Read the model definition and answer for the solid it produces. Units are mm, in the model's axes. Face numbers are marked on the shaded views. A direction names the side the tool comes from. Give positions to 0.01 mm unless a question says otherwise; leave off trailing zeros. Order: outer loops, then holes, each group sorted by start corner. A loop starts at its lowest first (then second) coordinate and runs counter-clockwise, first axis right, second up. Notation, with made-up numbers: (38.25, 86.5) - (67.25, 86.5) arc R18 ccw to (67.25, 93.5) - close; hole circle Ø4 at (64, -30). An arc over 180 degrees is marked (long way). Return JSON: item names as keys, results as strings.
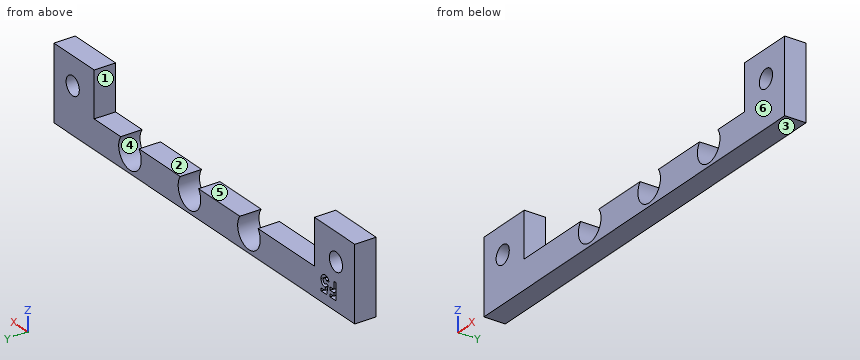
```python
from build123d import *

# Parameters (mm, degrees)
BOSS_EXTRUDE1_OUTLINE_R = 1.75
BOSS_EXTRUDE1_DEPTH     = 4
CUT_EXTRUDE1_DEPTH      = 1


# Read off the part's stored shape, not the designer's step: Boss-Extrude1
with BuildPart() as part:
    # Boss-Extrude1 outline → Boss-Extrude1 (new body)
    with BuildSketch(Plane(origin=(0, 0, 0), x_dir=(1, 0, 0), z_dir=(0, 1, 0))):
        with BuildLine():
            Line((24.976474615, -10.33744254), (35.92307775, -10.33744254))
            ThreePointArc((35.92307775, -10.33744254), (38.359776182, -5.587442326), (40.796474615, -10.33744254))
            Line((40.796474615, -10.33744254), (47.859776182, -10.33744254))
            Line((47.859776182, -10.33744254), (47.859776182, -18.81631662))
            Line((47.859776182, -18.81631662), (58.584776182, -18.81631662))
            Line((58.584776182, -18.81631662), (58.584776182, -4.977921711))
            Line((58.584776182, -4.977921711), (-21.415223818, -4.977921711))
            Line((-21.415223818, -4.977921711), (-21.415223818, -18.81631662))
            Line((-21.415223818, -18.81631662), (-10.690223818, -18.81631662))
            Line((-10.690223818, -18.81631662), (-10.690223818, -10.33744254))
            Line((-10.690223818, -10.33744254), (4.28307775, -10.33744254))
            ThreePointArc((4.28307775, -10.33744254), (6.719776183, -5.587442326), (9.156474615, -10.33744254))
            Line((9.156474615, -10.33744254), (20.10307775, -10.33744254))
            ThreePointArc((20.10307775, -10.33744254), (22.539776182, -5.587442326), (24.976474615, -10.33744254))
        make_face()
        with Locations((-16.415223818, -13.587442433)):
            Circle(BOSS_EXTRUDE1_OUTLINE_R, mode=Mode.SUBTRACT)
        with Locations((53.584776182, -13.587442433)):
            Circle(BOSS_EXTRUDE1_OUTLINE_R, mode=Mode.SUBTRACT)
    extrude(amount=BOSS_EXTRUDE1_DEPTH)

    # Sketch2 → Cut-Extrude1 (cut)
    with BuildSketch(Plane(origin=(0, 4, 0), x_dir=(1, 0, 0), z_dir=(0, 1, 0))):
        Polygon((-16.41198232, -6.812466594), (-14.865187448, -6.812466594), (-14.865187448, -7.382338389), (-15.842110525, -7.382338389), (-15.842110525, -7.992915312), (-14.865187448, -7.992915312), (-14.865187448, -8.562787107), (-15.842110525, -8.562787107), (-15.842110525, -9.987466594), (-16.41198232, -9.987466594), align=None)
        with BuildLine():
            Line((-13.949958082, -6.812466594), (-12.504290013, -6.812466594))
            Line((-12.504290013, -6.812466594), (-12.504290013, -7.341633261))
            Line((-12.504290013, -7.341633261), (-13.498385565, -7.341633261))
            Line((-13.498385565, -7.341633261), (-13.622409003, -7.942033902))
            add(Edge.make_bspline(
                [(-13.622409003, -7.942033902), (-13.605509034, -7.937327047), (-13.572178824, -7.928044162), (-13.52196682, -7.918734604), (-13.473304391, -7.912700444), (-13.441372402, -7.911895568), (-13.425879556, -7.911505055)],
                knots=[0, 0, 0, 0, 1.05461699, 2.079921384, 3.068411212, 4, 4, 4, 4], degree=3))
            add(Edge.make_bspline(
                [(-13.425879556, -7.911505055), (-13.392119021, -7.912278658), (-13.325569569, -7.913803601), (-13.228216166, -7.928280275), (-13.134994532, -7.951080599), (-13.046189934, -7.983598566), (-12.961889124, -8.025921539), (-12.881989912, -8.077120472), (-12.806394235, -8.137285289), (-12.73644499, -8.20645366), (-12.672172703, -8.282402096), (-12.616291615, -8.364548366), (-12.568565678, -8.451721144), (-12.530606118, -8.544462294), (-12.500645197, -8.642189339), (-12.478994766, -8.744964906), (-12.466191785, -8.852910799), (-12.464465382, -8.926554564), (-12.463584884, -8.96411423)],
                knots=[0, 0, 0, 0, 1.01440847, 1.999622559, 2.951875003, 3.895578053, 4.836219714, 5.782137149, 6.743708247, 7.735272588, 8.734977101, 9.730283169, 10.717124674, 11.717316708, 12.737475749, 13.78628267, 14.87096371, 16, 16, 16, 16], degree=3))
            add(Edge.make_bspline(
                [(-12.463584884, -8.96411423), (-12.464660866, -9.002100285), (-12.466784093, -9.077057875), (-12.480636202, -9.187272048), (-12.505085424, -9.292832343), (-12.538668877, -9.394021345), (-12.582912926, -9.490095338), (-12.63612245, -9.582049577), (-12.699197079, -9.669201514), (-12.771517834, -9.750657738), (-12.850139982, -9.82511029), (-12.93385401, -9.890606342), (-13.022071802, -9.94572074), (-13.114795487, -9.990262491), (-13.211493079, -10.025503132), (-13.312193927, -10.051156636), (-13.417387424, -10.065867495), (-13.488800141, -10.067862709), (-13.525098306, -10.06887685)],
                knots=[0, 0, 0, 0, 1.06808661, 2.107647099, 3.116961351, 4.110378221, 5.100014249, 6.085620622, 7.093190682, 8.119403071, 9.144090782, 10.133780668, 11.103064255, 12.062861538, 13.020824475, 13.992378307, 14.979551724, 16, 16, 16, 16], degree=3))
            add(Edge.make_bspline(
                [(-13.525098306, -10.06887685), (-13.557558674, -10.068047219), (-13.621577314, -10.066411014), (-13.715873961, -10.056354031), (-13.806786399, -10.038573192), (-13.893831984, -10.012839713), (-13.97792658, -9.981167676), (-14.058098031, -9.941555807), (-14.134786891, -9.894758372), (-14.207775393, -9.841629423), (-14.275877579, -9.781781722), (-14.338034038, -9.716268103), (-14.394621073, -9.645914331), (-14.444427811, -9.569852456), (-14.487298122, -9.488194854), (-14.525316388, -9.40190388), (-14.556434719, -9.310078379), (-14.572226377, -9.24641984), (-14.580251551, -9.214069158)],
                knots=[0, 0, 0, 0, 1.054957082, 2.080596141, 3.077793124, 4.061112343, 5.027190972, 5.994718051, 6.962465889, 7.943658696, 8.924948258, 9.904494768, 10.875059, 11.855380583, 12.854004648, 13.869083016, 14.917087635, 16, 16, 16, 16], degree=3))
            Line((-14.580251551, -9.214069158), (-13.9289695, -9.214069158))
            add(Edge.make_bspline(
                [(-13.9289695, -9.214069158), (-13.917064048, -9.236486864), (-13.893927162, -9.280053116), (-13.849915688, -9.337893862), (-13.800647638, -9.387217966), (-13.746567435, -9.428507334), (-13.687324675, -9.459440626), (-13.625333386, -9.482899003), (-13.559814799, -9.496454731), (-13.515193749, -9.498149331), (-13.492661407, -9.499005055)],
                knots=[0, 0, 0, 0, 1.104910296, 2.147267069, 3.153527244, 4.136738762, 5.099945312, 6.05603338, 7.018353, 8, 8, 8, 8], degree=3))
            add(Edge.make_bspline(
                [(-13.492661407, -9.499005055), (-13.476956667, -9.49841417), (-13.446057326, -9.497251594), (-13.400532034, -9.491101274), (-13.357076143, -9.479452707), (-13.315366568, -9.463322149), (-13.275291268, -9.443205522), (-13.237424734, -9.417809591), (-13.201108159, -9.388577933), (-13.166894426, -9.355034506), (-13.135906647, -9.317641387), (-13.108733754, -9.277459932), (-13.08443744, -9.235382981), (-13.066440789, -9.189743761), (-13.051703054, -9.141905074), (-13.040849589, -9.09150606), (-13.03436342, -9.038487855), (-13.033762974, -9.002293813), (-13.033456679, -8.983830777)],
                knots=[0, 0, 0, 0, 0.978869489, 1.925942215, 2.855067702, 3.774946051, 4.70828698, 5.642468714, 6.60995405, 7.609372294, 8.622401667, 9.629904756, 10.629323, 11.642352373, 12.678539694, 13.745912462, 14.850161547, 16, 16, 16, 16], degree=3))
            add(Edge.make_bspline(
                [(-13.033456679, -8.983830777), (-13.03381217, -8.965796309), (-13.034504141, -8.930691779), (-13.040228266, -8.879145756), (-13.050468615, -8.830237908), (-13.064421178, -8.783593638), (-13.082282125, -8.739496193), (-13.104109396, -8.697683084), (-13.129996239, -8.65836566), (-13.160081636, -8.622344386), (-13.192164393, -8.589304649), (-13.226631584, -8.560408358), (-13.263172677, -8.536426443), (-13.300652202, -8.515489534), (-13.340566208, -8.500252107), (-13.382017188, -8.489758654), (-13.424961552, -8.48205898), (-13.454252971, -8.481606596), (-13.469128755, -8.48137685)],
                knots=[0, 0, 0, 0, 1.166249705, 2.270133367, 3.348514167, 4.393962215, 5.415026464, 6.420877785, 7.440098956, 8.453121383, 9.451844239, 10.415694839, 11.355045125, 12.27538808, 13.187007209, 14.108269027, 15.039275622, 16, 16, 16, 16], degree=3))
            add(Edge.make_bspline(
                [(-13.469128755, -8.48137685), (-13.485287313, -8.481989978), (-13.51767253, -8.483218817), (-13.565788856, -8.493217552), (-13.613325034, -8.509399257), (-13.660545412, -8.531724482), (-13.706981248, -8.560941158), (-13.753858004, -8.59520897), (-13.799606617, -8.637017798), (-13.828694857, -8.668157109), (-13.843743138, -8.684266474)],
                knots=[0, 0, 0, 0, 0.88288272, 1.769486374, 2.674910571, 3.623812639, 4.617874466, 5.670434592, 6.794841017, 8, 8, 8, 8], degree=3))
            Line((-13.843743138, -8.684266474), (-14.323300429, -8.574235424))
            Line((-14.323300429, -8.574235424), (-13.949958082, -6.812466594))
        make_face()
    extrude(amount=-CUT_EXTRUDE1_DEPTH, mode=Mode.SUBTRACT)


solid = part.part
```
Q1. Given pin 1 (2 mm diameter, centred on x = 16.5, y = 2.5, fed in from +Z); pin 2 (5.5 mm diameter, centred on x = 38.36, z = 8.59, fed in from -Y), each flat-ended and moving along its own axis, determine where each tip first touches the part or whether it passes through.
Values:
{"pin 1": "stops at z = 10.34", "pin 2": "passes through"}
Q2. Determine the mould class of the marked faces 1, 2, 3 and 4 for opening direction Z: released by +Z, released by -Z, zero draft, split by the parting line, or undercut.
Values:
{"face 1": "zero draft", "face 2": "released by +Z", "face 3": "released by -Z", "face 4": "undercut"}
Q3. A cutting plane is placed at A-A (x = 28.5). Write down the section's boundary in (y, z), and give its area (3 significant figures).
Values:
{"outline": "(0, 4.98) - (4, 4.98) - (4, 10.34) - (0, 10.34) - close", "area": "21.4 mm²"}
Q4. For the marked faces 5 and 6, determine the directions among +Z, -Z, +X, -X, +Y, -Y from which every point of the face is accessible in a straight line to the end or side of a thin tool.
Values:
{"face 5": "+Z, +Y, -Y", "face 6": "+Z, -Z, +X, -X, -Y"}
Q5. A cutting plane is placed at B-B (y = 1.85). Write down the section's boundary in (x, z).
Values:
{"outline": "(-21.42, 4.98) - (58.58, 4.98) - (58.58, 18.82) - (47.86, 18.82) - (47.86, 10.34) - (40.8, 10.34) arc R3 cw (long way) to (35.92, 10.34) - (24.98, 10.34) arc R3 cw (long way) to (20.1, 10.34) - (9.16, 10.34) arc R3 cw (long way) to (4.28, 10.34) - (-10.69, 10.34) - (-10.69, 18.82) - (-21.42, 18.82) - close; hole circle Ø3.5 at (-16.42, 13.59); hole circle Ø3.5 at (53.58, 13.59)"}
Q6. Consider L1, parallel to X at y = 2.35, z = 7.5; L2, parallel to X at y = 2.1, z = 17.25; L3, parallel to X at y = 0.6, z = 13. Determine where each line is inside the solid, lowest interval first.
Values:
{"L1": "x = -21.42 to 3.92, 9.52 to 19.74, 25.34 to 35.56, 41.16 to 58.58", "L2": "x = -21.42 to -10.69, 47.86 to 58.58", "L3": "x = -21.42 to -18.06, -14.77 to -10.69, 47.86 to 51.94, 55.23 to 58.58"}
